Answer from the drawing. Dimensions are ordinates in mm from the lowest x, y and z of the part. A direction names the side the tool comes from. Give positions to 0.01 mm unless a question says otherwise; leave off trailing zeros. Order: outer loops, then holes, each group sorted by start corner. A loop starts at its lowest first (then second) coordinate and runs counter-clockwise, first axis right, second up. Notation, with made-up numbers: (22, 48) -> (61, 48) arc R37 cw to (61, 86) -> close; hole circle Ø2 at (32.5, -20.75). An arc over 180 degrees is marked (long way). Answer as a JSON object with one key per item and string values. Group by question number.
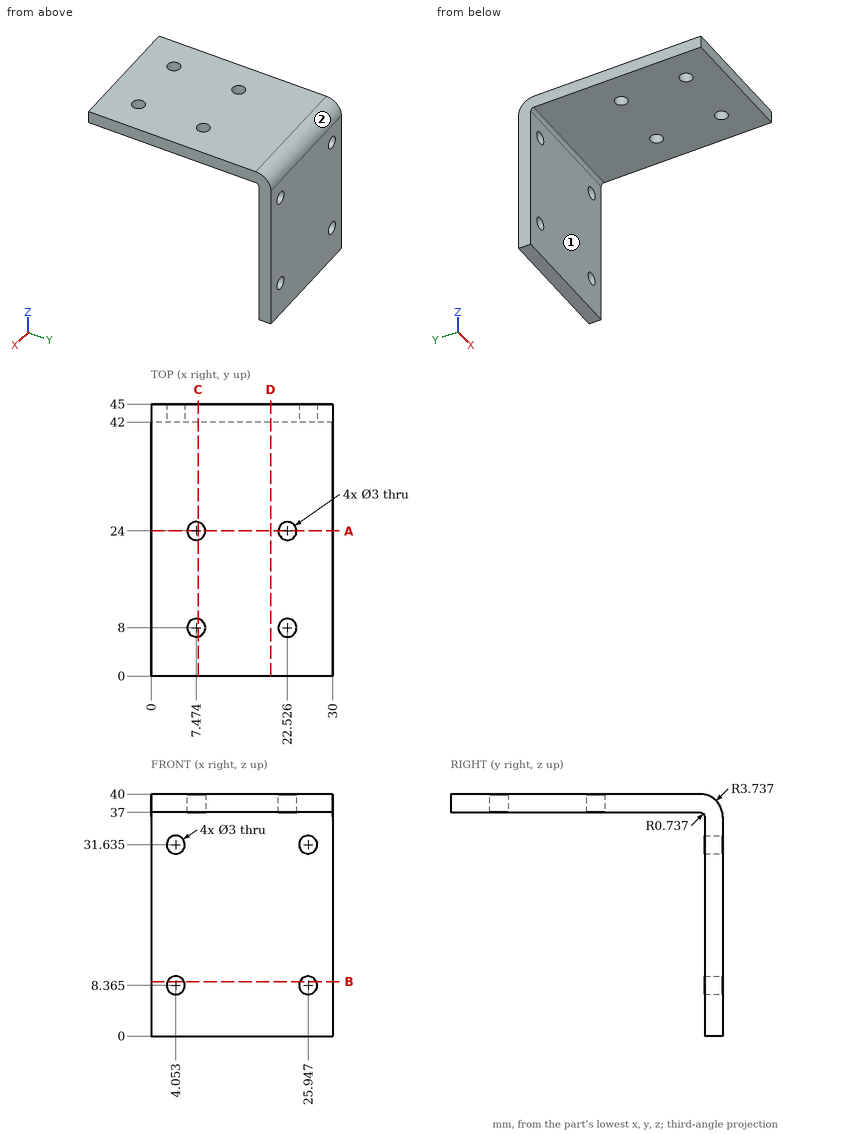
(1) A cutting plane is placed at D-D (x = 19.75). Determine the outline of the cut face in (y, z), and give its area (3 significant figures).
(2) Which of the six approach directions +Z, -Z, +X, -X, +Y, -Y give full straight-line access (tool end or side, diameter ignored) to the marked faces 1 and 2?
(3) Flat-ended cylindrical pins translate along their axes: pin 1 Ø6 at (x, z) = (10, 5.5) entering from -Y; pin 2 Ø4 at (x, y) = (22.53, 8) entering from +Z; pin 3 Ø15 at (x, y) = (18, 17) entering from -Z. Find the tip coordinate at first contact, or state that the pin passes through.
(4) A cutting plane is placed at B-B (z = 9). Determine the outline of the cut face in (x, y).
(5) Find the intervals of material crossed by line 1 along Y through (x, z) = (5.5, 13); line 2 along Y through (x, z) = (23.5, 38.5) (1 decimal); line 3 along Z through (x, y) = (21, 20.5), in increasing order. Write a range as [from, to].
(6) A cutting plane is placed at A-A (y = 24). Determine the outline of the cut face in (x, z) (1 decimal).
(7) A cutting plane is placed at C-C (x = 7.75). Determine the outline of the cut face in (y, z) (1 decimal).
Check sheet entries:
{
 "1": {"outline": "(0, 37) -> (41.26, 37) arc R0.74 cw to (42, 36.26) -> (42, 0) -> (45, 0) -> (45, 36.26) arc R3.74 ccw to (41.26, 40) -> (0, 40) -> close", "area": "243 mm2"},
 "2": {"face 1": "-Z, +X, -X, -Y", "face 2": "+Z, +X, -X, +Y"},
 "3": {"pin 1": "stops at y = 42", "pin 2": "stops at z = 40", "pin 3": "stops at z = 37"},
 "4": {"outline": "(0, 42) -> (2.69, 42) -> (2.69, 45) -> (0, 45) -> close; (5.41, 42) -> (24.59, 42) -> (24.59, 45) -> (5.41, 45) -> close; (27.31, 42) -> (30, 42) -> (30, 45) -> (27.31, 45) -> close"},
 "5": {"line 1": "y = [42, 45]", "line 2": "y = [0, 6.9], [9.1, 22.9], [25.1, 44.3]", "line 3": "z = [37, 40]"},
 "6": {"outline": "(0, 37) -> (6, 37) -> (6, 40) -> (0, 40) -> close; (9, 37) -> (21, 37) -> (21, 40) -> (9, 40) -> close; (24, 37) -> (30, 37) -> (30, 40) -> (24, 40) -> close"},
 "7": {"outline": "(0, 37) -> (6.5, 37) -> (6.5, 40) -> (0, 40) -> close; (9.5, 37) -> (22.5, 37) -> (22.5, 40) -> (9.5, 40) -> close; (25.5, 37) -> (41.3, 37) arc R0.7 cw to (42, 36.3) -> (42, 0) -> (45, 0) -> (45, 36.3) arc R3.7 ccw to (41.3, 40) -> (25.5, 40) -> close"}
}
